Drawing for the job (mm, zero at the part's lowest x, y, z). A direction names the side the tool comes from. Give positions to 0.01 mm unless a question says otherwise; leave off trailing zeros. Write each loop counter-clockwise with the first axis right and the second up, starting at its lowest first coordinate (ties: lowest second). Pieces come first, ordered by that corner, then holes.
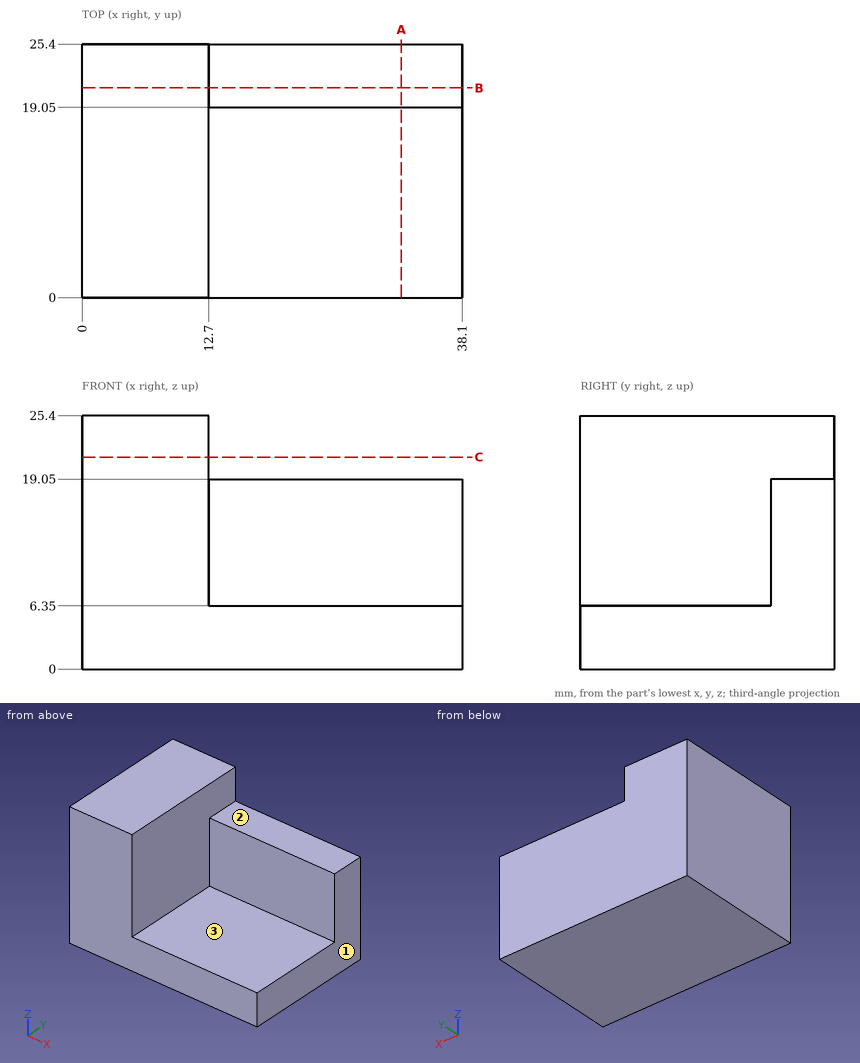
1. Slice it at B-B, the plane y = 21. Write the cut outline in (x, z).
Calculated:
outline: (0, 0) - (38.1, 0) - (38.1, 19.05) - (12.7, 19.05) - (12.7, 25.4) - (0, 25.4) - close
2. Slice it at A-A, the plane x = 32. Write the cut outline in (y, z).
Calculated:
outline: (0, 0) - (25.4, 0) - (25.4, 19.05) - (19.05, 19.05) - (19.05, 6.35) - (0, 6.35) - close
3. Slice it at C-C, the plane z = 21.25. Write the cut outline in (x, y).
Calculated:
outline: (0, 0) - (12.7, 0) - (12.7, 25.4) - (0, 25.4) - close
4. Which spindle directions (+Z, -Z, +X, -X, +Y, -Y) get a long thin tool onto all of the face, cutting with end or side? Do the marked faces 1, 2 and 3. Say none if no direction does.
Calculated:
face 1: +Z, -Z, +X, +Y, -Y
face 2: +Z, +X, +Y, -Y
face 3: +Z, +X, -Y
5. Pin check, flat tips, straight feed: P1, Ø6.5, axis at x = 30.5, z = 11, coming from the -Y side; P2, Ø5.5, axis at y = 8.5, z = 15.5, coming from the +X side; P3, Ø1.9, axis at x = 29.5, y = 21.5, coming from the +Z side. Stop position of each tip, or through.
Calculated:
P1: stops at y = 19.05
P2: stops at x = 12.7
P3: stops at z = 19.05
6. Probe probe 1 along X at (y, z) = (1.5, 21.75); probe 2 along Z at (x, y) = (33.5, 2); probe 3 along Z at (x, y) = (29, 19.75). List the from-to ranges inside material, lowest first.
Calculated:
probe 1: x = 0 to 12.7
probe 2: z = 0 to 6.35
probe 3: z = 0 to 19.05
